CAD build for the part. Positions are in the model's coordinates, mm. Give positions to 0.01 mm unless a question says otherwise; leave off trailing zeros. Loops run counter-clockwise (first coordinate to the right, second up) from the corner with the lowest first, then second, coordinate; pieces in that order, holes last. Notation, with made-up numbers: (67.5, 55) -> (87.5, 55) arc R23 cw to (87.5, 89) -> close; hole circle Ø10 at (-21, 54.5). An arc over 180 degrees is marked (long way). Use one line per item in the form item = value.
```python
from build123d import *

# Parameters (mm, degrees)
EXTRUDE_1_DEPTH        = 20
CHAMFER_1_SIZE         = 0.15
CHAMFER_2_SIZE2        = 0.3
CHAMFER_2_SIZE         = 0.214216777
CHAMFER_2_EDGE_2_SIZE2 = 0.214216777
CHAMFER_2_EDGE_2_SIZE  = 0.3


with BuildPart() as part:
    # Эскиз1 → Вытянуть1 (new body)
    with BuildSketch(Plane(origin=(0, 0, 0), x_dir=(1, 0, 0), z_dir=(0, 1, 0))):
        Polygon((11.981509397, 15.9), (21.372526833, 15.9), (9.391017436, 0), (0, 0), align=None)
    extrude(amount=EXTRUDE_1_DEPTH)

    # Фаска1
    chamfer_1_edges = [part.edges().sort_by_distance(p)[0] for p in [
        (15.381772134, 20, -7.95),
        (16.677018115, 20, -15.9),
        (5.990754698, 20, -7.95),
        (16.677018115, 0, -15.9),
        (15.381772134, 0, -7.95),
        (4.695508718, 0, 0),
        (5.990754698, 0, -7.95),
        (4.695508718, 20, 0),
    ]]
    chamfer(chamfer_1_edges, length=CHAMFER_1_SIZE)

    # Фаска2
    chamfer_2_edges = [part.edges().sort_by_distance(p)[0] for p in [
        (21.372526833, 10, -15.9),
    ]]
    chamfer(chamfer_2_edges, length=CHAMFER_2_SIZE, length2=CHAMFER_2_SIZE2)

    # Фаска2 edge 2
    chamfer_2_edge_2_edges = [part.edges().sort_by_distance(p)[0] for p in [
        (0, 10, 0),
    ]]
    chamfer(chamfer_2_edge_2_edges, length=CHAMFER_2_EDGE_2_SIZE, length2=CHAMFER_2_EDGE_2_SIZE2)


solid = part.part
```
1. Cut at B-B, the plane y = 5.75. Write the cut outline in (x, z), then the cut area to 3 significant figures.
Result sheet:
outline = (0.18, -0.24) -> (11.98, -15.9) -> (21.16, -15.9) -> (21.19, -15.66) -> (9.39, 0) -> (0.21, 0) -> close
area = 149 mm^2
2. Drop flat-ended pins along their axis: P1, Ø5, axis at x = 18.5, z = -4.5, coming from the -Y side; P2, Ø1.5, axis at y = 6.5, z = -4, coming from the +X side; P3, Ø6, axis at x = 10.5, y = 14.5, coming from the +Z side; P4, Ø8, axis at y = 16, z = -12, coming from the -X side. Give the stop position or say it passes through.
Result sheet:
P1 = through
P2 = 12.97
P3 = 0
P4 = 6.03
3. Cut at C-C, the plane z = -13.25. Write the cut outline in (x, y).
Result sheet:
outline = (9.98, 0.15) -> (10.17, 0) -> (19.19, 0) -> (19.38, 0.15) -> (19.38, 19.85) -> (19.19, 20) -> (10.17, 20) -> (9.98, 19.85) -> close
4. Cut at A-A, the plane x = 5.75. Write the cut outline in (y, z).
Result sheet:
outline = (0, -7.38) -> (0.15, -7.63) -> (19.85, -7.63) -> (20, -7.38) -> (20, -0.15) -> (19.85, 0) -> (0.15, 0) -> (0, -0.15) -> close
5. Drill centre lines: line 1 (X direction, y = 12.5, z = -2.5); line 2 (X direction, y = 15.25, z = -14.75); line 3 (Z direction, x = 11.5, y = 4.75). Where is each one in solid material? Low to high.
Result sheet:
line_1 = 1.88 to 11.27
line_2 = 11.11 to 20.51
line_3 = -15.26 to -2.8
